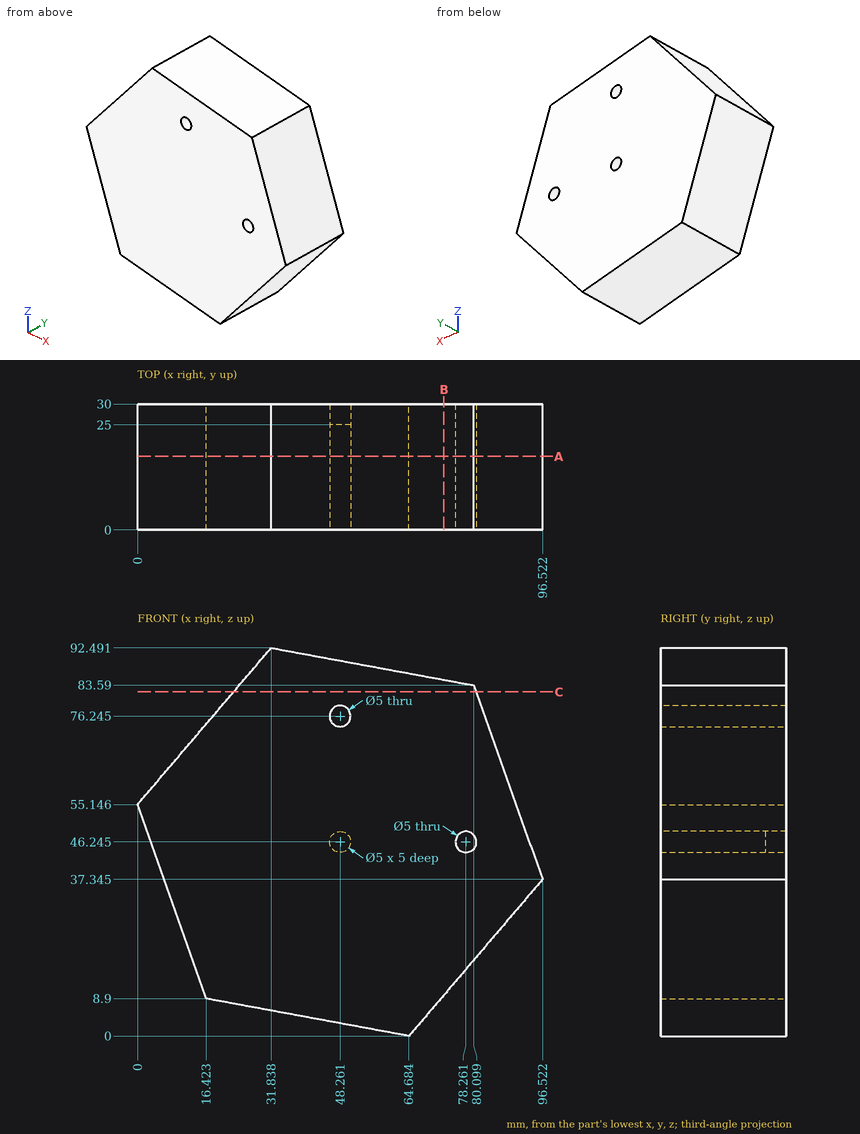
Job drawing, mm, ordinate dimensions from the low corner. One solid piece. Round coordinates to 2 decimals unless told otherwise and drop trailing zeros. Order: outer loops, then holes, each group sorted by start corner. A loop starts at its lowest first (then second) coordinate and runs counter-clockwise, first axis right, second up. Notation, with made-up numbers: M 89.25,-26 L 146.25,-26 A29 cw 146.25,-6 Z; hole C 6.25,63 d7. An arc over 180 degrees is marked long. Write each question's results on one line, items separated by ' | '. Start each with the question number.
(1) Drop flat-ended pins along their axis: pin 1 (4 mm diameter, centred on x = 18, z = 58.5, fed in from -Y); pin 2 (6 mm diameter, centred on y = 8.5, z = 61.5, fed in from +X); pin 3 (5 mm diameter, centred on y = 14, z = 18.5, fed in from +X); pin 4 (4.5 mm diameter, centred on x = 48.26, z = 76.25, fed in from -Y) (1 decimal). Give the stop position or say it passes through.
(2) Saw through at B-B, the plane x = 73. Give the cut face in (y, z) (1 decimal).
(3) Saw through at A-A, the plane y = 17.5. Give the cut face in (x, z) (1 decimal), then the cut area to 3 significant figures.
(4) Saw through at C-C, the plane z = 82. Give the cut face in (x, y) (1 decimal).
(5) Probe probe 1 along Z at (x, y) = (47, 3.5) (1 decimal); probe 2 along Z at (x, y) = (28, 10.75) (1 decimal); probe 3 along Z at (x, y) = (38, 13.25) (1 decimal). List the from-to ranges inside material, lowest first. Write a range as from..to.
Established:
1) pin 1: stops at y = 0 | pin 2: stops at x = 89.01 | pin 3: stops at x = 82.59 | pin 4: passes through
2) outline: M 0,9.8 L 30,9.8 L 30,84.9 L 0,84.9 Z
3) outline: M 0,55.1 L 16.4,8.9 L 64.7,0 L 96.5,37.3 L 80.1,83.6 L 31.8,92.5 Z; hole C 48.3,76.2 d5; hole C 78.3,46.2 d5 | area: 6,220 mm^2
4) outline: M 22.9,0 L 80.7,0 L 80.7,30 L 22.9,30 Z
5) probe 1: z = 3.3..74.1, 78.4..89.7 | probe 2: z = 6.8..88 | probe 3: z = 4.9..91.4
